```python
from build123d import *

# Parameters (mm, degrees)
F0_W     = 120
F0_H     = 150
F1_DEPTH = 60
F2_T     = -2.5
F3_W     = 7.0065811276
F3_H     = 60
F3_W_2   = 14.9013146758
F4_DEPTH = 25
F5_W     = 23.38815853
F5_H     = 60
F6_DEPTH = 25


with BuildPart() as f1:
    # F0 (on Top) → F1 (new body)
    with BuildSketch(Plane.XY):
        Rectangle(F0_W, F0_H)
    extrude(amount=F1_DEPTH)

    # F2
    f2_openings = [f1.faces().sort_by_distance(p)[0] for p in [
        (0, 0, 60),
    ]]
    offset(amount=F2_T, openings=f2_openings)

    # F3 (on face) → F4 (cut)
    with BuildSketch(Plane.YZ.offset(60)):
        with Locations((-78.5032905638, 30)):
            Rectangle(F3_W, F3_H)
        with Locations((-67.5493426621, 30)):
            Rectangle(F3_W_2, F3_H)
    extrude(amount=-F4_DEPTH, mode=Mode.SUBTRACT)

    # F5 (on face) → F6 (cut)
    with BuildSketch(Plane.YZ.offset(60)):
        with Locations((-11.694079265, 30)):
            Rectangle(F5_W, F5_H)
    extrude(amount=-F6_DEPTH, mode=Mode.SUBTRACT)


solid = f1.part
```
Part model, mm, in its own coordinate system. A direction names the side the tool comes from. Round coordinates to 2 decimals unless told otherwise and drop trailing zeros. Order: outer loops, then holes, each group sorted by start corner. A loop starts at its lowest first (then second) coordinate and runs counter-clockwise, first axis right, second up. Notation, with made-up numbers: M -11,25.5 L 25,25.5 A30 cw 25,60.5 Z; hole C 44,-37 d3. An arc over 180 degrees is marked long. Answer in a Markdown table with one row per item. Add a question column.
Q1. Cut at C-C on y = -62.5. Give the cut face in (x, z), and give its area (3 significant figures).
Q2. Pin check, flat tips, straight feed: pin 1 (1.5 mm diameter, centred on x = 1.5, y = -16.5, fed in from +Z); pin 2 (12 mm diameter, centred on y = -68.5, z = 36, fed in from +X); pin 3 (12.5 mm diameter, centred on x = 52.5, z = 43.5, fed in from -Y). Stop position of each tip, or through.
Q3. Wall check: L1, parallel to X at y = -37, z = 13.5; L2, parallel to Y at x = 13.5, z = 4.5; L3, parallel to Z at x = -14, y = -27. Give the ranges that are in metal, low to high. Write a range as from..to.
Q4. 3-axis set-ups, long thin cutter, end or side, ignore diameter. For faces 5 (the face through (57.5, 36, 31)), 6 (the face through (58, -60.099, 23)), 7 (the face through (-1, 1, 2.5)), 8 (the face through (-12, -72.5, 31)), 9 (the face through (58, 0, 23)): which of +Z, -Z, +X, -X, +Y, -Y reach the whole face in a straight line?
Q5. Cut at B-B on x = 49. Give the cut face in (y, z).
Q6. Mould opens along X. For faces 1 (the face through (-60, -1, 30)), 2 (the face through (57.5, -42, 31)), 3 (the face through (-1, 72.5, 31)), 4 (the face through (58, -23.388, 23)) say: +X half, -X half, draft (parallel to the pull), parting line (faces both ways), or undercut.
Q7. Cut at D-D on x = -44.5. Give the cut face in (y, z), and give its area (4 significant figures).
Q8. Cut at A-A on z = 10. Give the cut face in (x, y), and give its area (3 significant figures).
Established:
| question | item | result |
|---|---|---|
| 1 | outline | M -60,0 L 35,0 L 35,2.5 L -57.5,2.5 L -57.5,60 L -60,60 Z |
| 1 | area | 381 mm2 |
| 2 | pin 1 | stops at z = 2.5 |
| 2 | pin 2 | stops at x = 35 |
| 2 | pin 3 | stops at y = -60.1 |
| 3 | L1 | x = -60..-57.5, 57.5..60 |
| 3 | L2 | y = -75..-72.5, 72.5..75 |
| 3 | L3 | z = 0..2.5 |
| 4 | face 5 | +Z, -Y |
| 4 | face 6 | +Z, -Z, +X, -Y |
| 4 | face 7 | +Z |
| 4 | face 8 | +Z, +X |
| 4 | face 9 | +Z, -Z, +X |
| 5 | outline | M -60.1,0 L -23.39,0 L -23.39,2.5 L -60.1,2.5 Z; M 0,0 L 75,0 L 75,60 L 72.5,60 L 72.5,2.5 L 0,2.5 Z |
| 6 | face 1 | -X half |
| 6 | face 2 | undercut |
| 6 | face 3 | undercut |
| 6 | face 4 | draft |
| 7 | outline | M -75,0 L 75,0 L 75,60 L 72.5,60 L 72.5,2.5 L -72.5,2.5 L -72.5,60 L -75,60 Z |
| 7 | area | 662.5 mm2 |
| 8 | outline | M -60,-75 L 35,-75 L 35,-72.5 L -57.5,-72.5 L -57.5,72.5 L 57.5,72.5 L 57.5,0 L 60,0 L 60,75 L -60,75 Z; M 57.5,-60.1 L 60,-60.1 L 60,-23.39 L 57.5,-23.39 Z |
| 8 | area | 1,170 mm2 |
